from build123d import *

# Parameters (mm, degrees)
F0_W     = 180
F0_H     = 180
F1_DEPTH = 5
F3_DEPTH = 5


with BuildPart() as f1:
    # F0 (on Top) → F1 (new body)
    with BuildSketch(Plane.XY):
        Rectangle(F0_W, F0_H)
    extrude(amount=F1_DEPTH)

    # F2 (on face) → F3 (join)
    with BuildSketch(Plane.XY.offset(5)):
        with BuildLine():
            add(Edge.make_bspline(
                [(-84.6410161514, 90), (-90, 71.4359353945), (-90, 50)],
                knots=[4.1887902048, 4.1887902048, 4.1887902048, 4.7123889804, 4.7123889804, 4.7123889804], degree=2, weights=[1, 0.9659258263, 1]))
            Line((-84.6410161514, 90), (-90, 90))
            Line((-90, 90), (-90, 50))
        make_face()
        with BuildLine():
            add(Edge.make_bspline(
                [(-11.2701665379, 70), (-12.6331056415, 80.5572809), (-15.3589838486, 90)],
                knots=[1.8234765819, 1.8234765819, 1.8234765819, 2.0943951024, 2.0943951024, 2.0943951024], degree=2, weights=[1, 0.9908394147, 1]))
            Line((-15.3589838486, 90), (-84.6410161514, 90))
            add(Edge.make_bspline(
                [(-84.6410161514, 90), (-90, 71.4359353945), (-90, 50)],
                knots=[4.1887902048, 4.1887902048, 4.1887902048, 4.7123889804, 4.7123889804, 4.7123889804], degree=2, weights=[1, 0.9659258263, 1]))
            add(Edge.make_bspline(
                [(-90, 50), (-90, 3.8119784648), (-70, -19.2820323028)],
                knots=[4.7123889804, 4.7123889804, 4.7123889804, 5.7595865316, 5.7595865316, 5.7595865316], degree=2, weights=[1, 0.8660254038, 1]))
            Line((-70, -19.2820323028), (-70, 70))
            Line((-70, 70), (-11.2701665379, 70))
        make_face()
        with BuildLine():
            add(Edge.make_bspline(
                [(8.7877538268, 70), (7.5221386644, 80.333704529), (4.9909083395, 90)],
                knots=[4.9137469012, 4.9137469012, 4.9137469012, 5.1239058265, 5.1239058265, 5.1239058265], degree=2, weights=[1, 0.9944842314, 1]))
            Line((4.9909083395, 90), (-15.3589838486, 90))
            add(Edge.make_bspline(
                [(-11.2701665379, 70), (-12.6331056415, 80.5572809), (-15.3589838486, 90)],
                knots=[1.8234765819, 1.8234765819, 1.8234765819, 2.0943951024, 2.0943951024, 2.0943951024], degree=2, weights=[1, 0.9908394147, 1]))
            Line((-11.2701665379, 70), (8.7877538268, 70))
        make_face()
        with BuildLine():
            Line((90, 37.267799625), (90, 90))
            Line((90, 90), (4.9909083395, 90))
            add(Edge.make_bspline(
                [(8.7877538268, 70), (7.5221386644, 80.333704529), (4.9909083395, 90)],
                knots=[4.9137469012, 4.9137469012, 4.9137469012, 5.1239058265, 5.1239058265, 5.1239058265], degree=2, weights=[1, 0.9944842314, 1]))
            Line((8.7877538268, 70), (70, 70))
            Line((70, 70), (70, 47.1404520791))
            add(Edge.make_bspline(
                [(90, 37.267799625), (81.1696311978, 43.8495679277), (70, 47.1404520791)],
                knots=[3.9826613242, 3.9826613242, 3.9826613242, 4.3725520709, 4.3725520709, 4.3725520709], degree=2, weights=[1, 0.9810582529, 1]))
        make_face()
        with BuildLine():
            Line((90, -2.944e-07), (90, 37.267799625))
            add(Edge.make_bspline(
                [(90, 37.267799625), (81.1696311978, 43.8495679277), (70, 47.1404520791)],
                knots=[3.9826613242, 3.9826613242, 3.9826613242, 4.3725520709, 4.3725520709, 4.3725520709], degree=2, weights=[1, 0.9810582529, 1]))
            Line((70, 47.1404520791), (70, 25.9807621135))
            add(Edge.make_bspline(
                [(90, -2.944e-07), (90.0000002266, 17.3205079775), (70, 25.9807621135)],
                knots=[3.1415926438, 3.1415926438, 3.1415926438, 4.1887902048, 4.1887902048, 4.1887902048], degree=2, weights=[1, 0.8660254013, 1]))
        make_face()
        with BuildLine():
            add(Edge.make_bspline(
                [(70, -25.9807621135), (89.9999997734, -17.3205081738), (90, -2.944e-07)],
                knots=[2.0943951024, 2.0943951024, 2.0943951024, 3.1415926438, 3.1415926438, 3.1415926438], degree=2, weights=[1, 0.8660254062, 1]))
            add(Edge.make_bspline(
                [(90, -2.944e-07), (90.0000002266, 17.3205079775), (70, 25.9807621135)],
                knots=[3.1415926438, 3.1415926438, 3.1415926438, 4.1887902048, 4.1887902048, 4.1887902048], degree=2, weights=[1, 0.8660254013, 1]))
            Line((70, 25.9807621135), (70, -25.9807621135))
        make_face()
        with BuildLine():
            Line((90, -37.267799625), (90, -2.944e-07))
            add(Edge.make_bspline(
                [(70, -25.9807621135), (89.9999997734, -17.3205081738), (90, -2.944e-07)],
                knots=[2.0943951024, 2.0943951024, 2.0943951024, 3.1415926438, 3.1415926438, 3.1415926438], degree=2, weights=[1, 0.8660254062, 1]))
            Line((70, -25.9807621135), (70, -47.1404520791))
            add(Edge.make_bspline(
                [(70, -47.1404520791), (81.1696311978, -43.8495679277), (90, -37.267799625)],
                knots=[1.9106332362, 1.9106332362, 1.9106332362, 2.300523983, 2.300523983, 2.300523983], degree=2, weights=[1, 0.9810582529, 1]))
        make_face()
        with BuildLine():
            Line((-90, 50), (-90, -24.53559925))
            add(Edge.make_bspline(
                [(-90, -24.53559925), (-81.1696311978, -37.6991358555), (-70, -44.2809041582)],
                knots=[2.4118649974, 2.4118649974, 2.4118649974, 2.8017557441, 2.8017557441, 2.8017557441], degree=2, weights=[1, 0.9810582529, 1]))
            Line((-70, -44.2809041582), (-70, -19.2820323028))
            add(Edge.make_bspline(
                [(-90, 50), (-90, 3.8119784648), (-70, -19.2820323028)],
                knots=[4.7123889804, 4.7123889804, 4.7123889804, 5.7595865316, 5.7595865316, 5.7595865316], degree=2, weights=[1, 0.8660254038, 1]))
        make_face()
        with BuildLine():
            add(Edge.make_bspline(
                [(9.4810733311, 36.876450834), (10, 43.4097265114), (10, 50)],
                knots=[4.5807738328, 4.5807738328, 4.5807738328, 4.7123889804, 4.7123889804, 4.7123889804], degree=2, weights=[1, 0.9978354629, 1]))
            Line((10, 50), (0, 50))
            Line((0, 50), (0, 30))
            Line((0, 30), (-11.2701665379, 30))
            add(Edge.make_bspline(
                [(-50, -30), (-19.0161332303, -30), (-11.2701665379, 30)],
                knots=[0, 0, 0, 1.3181160717, 1.3181160717, 1.3181160717], degree=2, weights=[1, 0.790569415, 1]))
            Line((-50, -30), (-50, -50))
            add(Edge.make_bspline(
                [(-50, -50), (-23.7994473959, -50), (-5.9908211975, -17.9704221034)],
                knots=[3.1415926536, 3.1415926536, 3.1415926536, 3.9650296719, 3.9650296719, 3.9650296719], degree=2, weights=[1, 0.9164344551, 1]))
            add(Edge.make_bspline(
                [(9.4810733311, 36.876450834), (-20.6970548218, 13.8493839138), (-5.9908211975, -17.9704221034)],
                knots=[5.4537813034, 5.4537813034, 5.4537813034, 6.6508192072, 6.6508192072, 6.6508192072], degree=2, weights=[1, 0.8261709721, 1]))
        make_face()
        with BuildLine():
            Line((0, 50), (-10, 50))
            add(Edge.make_bspline(
                [(-11.2701665379, 30), (-10, 39.8386676966), (-10, 50)],
                knots=[1.3181160717, 1.3181160717, 1.3181160717, 1.5707963268, 1.5707963268, 1.5707963268], degree=2, weights=[1, 0.9920296963, 1]))
            Line((-11.2701665379, 30), (0, 30))
            Line((0, 30), (0, 50))
        make_face()
        with BuildLine():
            add(Edge.make_bspline(
                [(-11.2701665379, 30), (-10, 39.8386676966), (-10, 50)],
                knots=[1.3181160717, 1.3181160717, 1.3181160717, 1.5707963268, 1.5707963268, 1.5707963268], degree=2, weights=[1, 0.9920296963, 1]))
            Line((-10, 50), (-50, 50))
            Line((-50, 50), (-50, 30))
            Line((-50, 30), (-11.2701665379, 30))
        make_face()
        with BuildLine():
            Line((50, 30), (50, 50))
            add(Edge.make_bspline(
                [(50, 50), (26.6801438826, 50), (9.4810733311, 36.876450834)],
                knots=[4.7123889804, 4.7123889804, 4.7123889804, 5.4537813034, 5.4537813034, 5.4537813034], degree=2, weights=[1, 0.932075377, 1]))
            add(Edge.make_bspline(
                [(-5.9908211975, -17.9704221034), (6.9772353101, 5.3531836285), (9.4810733311, 36.876450834)],
                knots=[3.9650296719, 3.9650296719, 3.9650296719, 4.5807738328, 4.5807738328, 4.5807738328], degree=2, weights=[1, 0.9529805535, 1]))
            add(Edge.make_bspline(
                [(-5.9908211975, -17.9704221034), (8.8123631833, -50), (50, -50)],
                knots=[0.3676339, 0.3676339, 0.3676339, 1.5707963268, 1.5707963268, 1.5707963268], degree=2, weights=[1, 0.8244417633, 1]))
            Line((50, -50), (50, -30))
            add(Edge.make_bspline(
                [(10, 0), (10, -30), (50, -30)],
                knots=[0, 0, 0, 1.5707963268, 1.5707963268, 1.5707963268], degree=2, weights=[1, 0.7071067812, 1]))
            add(Edge.make_bspline(
                [(50, 30), (10, 30), (10, 0)],
                knots=[4.7123889804, 4.7123889804, 4.7123889804, 6.2831853072, 6.2831853072, 6.2831853072], degree=2, weights=[1, 0.7071067812, 1]))
        make_face()
        with BuildLine():
            add(Edge.make_bspline(
                [(-5.9908211975, -17.9704221034), (6.9772353101, 5.3531836285), (9.4810733311, 36.876450834)],
                knots=[3.9650296719, 3.9650296719, 3.9650296719, 4.5807738328, 4.5807738328, 4.5807738328], degree=2, weights=[1, 0.9529805535, 1]))
            add(Edge.make_bspline(
                [(9.4810733311, 36.876450834), (-20.6970548218, 13.8493839138), (-5.9908211975, -17.9704221034)],
                knots=[5.4537813034, 5.4537813034, 5.4537813034, 6.6508192072, 6.6508192072, 6.6508192072], degree=2, weights=[1, 0.8261709721, 1]))
        make_face()
        with BuildLine():
            Line((90, -90), (90, -37.267799625))
            add(Edge.make_bspline(
                [(70, -47.1404520791), (81.1696311978, -43.8495679277), (90, -37.267799625)],
                knots=[1.9106332362, 1.9106332362, 1.9106332362, 2.300523983, 2.300523983, 2.300523983], degree=2, weights=[1, 0.9810582529, 1]))
            Line((70, -47.1404520791), (70, -70))
            Line((70, -70), (-70, -70))
            Line((-70, -70), (-70, -44.2809041582))
            add(Edge.make_bspline(
                [(-90, -24.53559925), (-81.1696311978, -37.6991358555), (-70, -44.2809041582)],
                knots=[2.4118649974, 2.4118649974, 2.4118649974, 2.8017557441, 2.8017557441, 2.8017557441], degree=2, weights=[1, 0.9810582529, 1]))
            Line((-90, -24.53559925), (-90, -90))
            Line((-90, -90), (90, -90))
        make_face()
    extrude(amount=F3_DEPTH)


solid = f1.part
Can you work these out from the model? Positions are in its coordinate system, mm. A direction names the side the tool comes from. Give positions to 0.01 mm unless a question says otherwise; leave off trailing zeros. Loops run counter-clockwise (first coordinate to the right, second up) from the corner with the lowest first, then second, coordinate; pieces in that order, holes last. Notation, with made-up numbers: (15.5, 55.5) -> (22.5, 55.5) arc R25 cw to (22.5, 81.5) -> close; hole circle Ø11 at (32, 12). An arc over 180 degrees is marked (long way). Use one line per item in the form item = value.
1) If we section it at B-B (z = 8.25): Count the separate pieces of the cut face and the enclosed holes in it, plus the area to 3 significant figures.
Answers:
separate_pieces = 2
enclosed_holes = 1
area = 18,100 mm²
2) For faces 1 (the face through (50, -40, 7)), 2 (the face through (1, 90, 5)), which set-ups out of +Z, -Z, +X, -X, +Y, -Y let a thin tool reach every point of the face, with its end or its side?
Answers:
face_1 = +Z
face_2 = +Z, -Z, +X, -X, +Y
3) I need wall thicknesses on line 1 along Y through (x, z) = (50.5, 8); line 2 along X through (y, z) = (-41, 5.25). Which ranges of each line are inside material? Lowest first, please.
Answers:
line_1 = -90 to -70, 70 to 90
line_2 = -90 to -70, -50 to -25.12, 15.66 to 50, 70 to 90
4) Will this pin go through, and if not, where does the flat tip stop? pin 1 (2 mm diameter, centred on x = 58.5, y = 59, fed in from +Z).
Answers:
pin_1 = 5
5) If we section it at A-A (y = 62): Please give me the cut outline in (x, z), plus the area to 3 significant figures.
Answers:
outline = (-90, 0) -> (90, 0) -> (90, 10) -> (70, 10) -> (70, 5) -> (-70, 5) -> (-70, 10) -> (-90, 10) -> close
area = 1,100 mm²
6) We'd pull the mould along X, two halves only. Please class faces 3 (the face through (90, -1, 5)), 4 (the face through (-1, -90, 5)), 5 (the face through (70, 1, 7)): released by +X, released by -X, zero draft, split by the parting line, or undercut.
Answers:
face_3 = released by +X
face_4 = zero draft
face_5 = undercut
